Input: part model. Units: mm. Frame: model coordinates. A direction names the side the tool comes from. Coordinates: 2 decimals unless noted, no trailing zeros. Loops run counter-clockwise (first coordinate to the right, second up) from the corner with the lowest first, then second, coordinate; pieces in that order, holes last. Notation, with made-up numbers: (-38.75, 80.5) -> (16.25, 80.5) arc R10 ccw to (16.25, 88.5) -> close; hole circle Ø1 at (35.25, -38). An arc over 180 degrees is marked (long way). Put each result on its own line as item: value. Start each with the question number.
1) Cut plane A-A (y = -8). Return the cut outline in (x, z).
2) Contact query for flat-ended pins moving along their axis: P1, Ø2.5, axis at y = -6.5, z = 94, coming from the -X side; P2, Ø20, axis at x = 64.5, z = 92, coming from the -Y side; P3, Ø2, axis at x = 71.5, y = -8.5, coming from the +Z side; P4, Ø4, axis at y = -8, z = 77, coming from the -X side. Output: stop coordinate, or through.
3) Material intervals for L1, parallel to X at y = -7.4, z = 60; L2, parallel to X at y = -7.75, z = 94; L3, parallel to Y at x = 115.5, z = 38, sorted ascending.
4) Cut plane B-B (z = 69). Return the cut outline in (x, y), plus the area to 3 significant figures.
5) Cut plane C-C (x = 55.5). Return the cut outline in (y, z).
6) Set-up query: faces 1 (the flat face through (61.25, -6, 117)), 2 (the flat face through (64, -7, 112)), 3 (the flat face through (91, -2, 120)). Return all of +Z, -Z, +X, -X, +Y, -Y with unobstructed straight access to the full face (end or side cutting, diameter ignored); none if empty.
7) Pull-direction query (X, two-part tool) for faces 4 (the flat face through (0, -2, 61)), 5 (the flat face through (56, -7, 112)), 6 (the cylindrical face through (61, -8, 1)); classes: pulls with the +X half, pulls with the -X half, needs draft (parallel to the pull), parting line crosses it, or undercut.
from build123d import *

# Parameters (mm, degrees)
F1_DEPTH = 5
F2_DEPTH = 10
F3_R     = 5


with BuildPart() as f1:
    # F0 (on Front) → F1 (new body)
    with BuildSketch(Plane.XZ):
        with BuildLine():
            Line((54, 60), (54, 79.078784))
            ThreePointArc((54, 79.078784), (48.16784, 43.875485), (80, 60))
            ThreePointArc((80, 60), (76.124515, 71.83216), (66, 79.078784))
            Line((66, 79.078784), (66, 60))
            Line((66, 60), (60, 60))
            Line((60, 60), (54, 60))
        make_face()
        with BuildLine():
            ThreePointArc((60, 80), (56.964846, 79.768355), (54, 79.078784))
            Line((54, 79.078784), (54, 60))
            Line((54, 60), (60, 60))
            Line((60, 60), (66, 60))
            Line((66, 60), (66, 79.078784))
            ThreePointArc((66, 79.078784), (63.035154, 79.768355), (60, 80))
        make_face()
        with BuildLine():
            Line((60, 80), (54, 80))
            Line((54, 80), (54, 79.078784))
            ThreePointArc((54, 79.078784), (56.964846, 79.768355), (60, 80))
        make_face()
        with BuildLine():
            Line((66, 79.078784), (66, 80))
            Line((66, 80), (60, 80))
            ThreePointArc((60, 80), (63.035154, 79.768355), (66, 79.078784))
        make_face()
        Polygon((58.75, 112), (54, 112), (54, 80), (60, 80), (66, 80), (66, 112), (61.25, 112), (61.25, 117.5), (58.75, 117.5), align=None)
    extrude(amount=F1_DEPTH)

    # F0 (on Front) → F2 (join)
    with BuildSketch(Plane.XZ):
        with BuildLine():
            Line((0, 120), (0, 0))
            Line((0, 0), (120, 0))
            Line((120, 0), (120, 120))
            Line((120, 120), (66, 120))
            Line((66, 120), (66, 112))
            Line((66, 112), (66, 80))
            Line((66, 80), (66, 79.078784))
            ThreePointArc((66, 79.078784), (76.124515, 71.83216), (80, 60))
            ThreePointArc((80, 60), (48.16784, 43.875485), (54, 79.078784))
            Line((54, 79.078784), (54, 80))
            Line((54, 80), (54, 112))
            Line((54, 112), (54, 120))
            Line((54, 120), (0, 120))
        make_face()
        Polygon((58.75, 120), (54, 120), (54, 112), (58.75, 112), (58.75, 117.5), align=None)
        Polygon((66, 112), (66, 120), (61.25, 120), (61.25, 117.5), (61.25, 112), align=None)
    extrude(amount=F2_DEPTH)

    # F3
    f3_edges = [f1.edges().sort_by_distance(p)[0] for p in [
        (0, -10, 60),
        (60, -10, 0),
        (120, -10, 60),
        (90.625, -10, 120),
        (29.375, -10, 120),
    ]]
    fillet(f3_edges, radius=F3_R)


solid = f1.part
Results found:
1. outline: (1, 1) -> (119, 1) -> (119, 119) -> (61.25, 119) -> (61.25, 112) -> (66, 112) -> (66, 79.08) arc R20 cw (long way) to (54, 79.08) -> (54, 112) -> (58.75, 112) -> (58.75, 119) -> (1, 119) -> close
2. P1: stops at x = 0.01
2. P2: stops at y = -10
2. P3: stops at z = 119.33
2. P4: stops at x = 0.1
3. L1: x = 0.61 to 40, 80 to 119.39
3. L2: x = 0.82 to 54, 66 to 119.18
3. L3: y = -9.97 to 0
4. outline: (0, -5) arc R5 ccw to (5, -10) -> (42.14, -10) -> (42.14, -5) -> (77.86, -5) -> (77.86, -10) -> (115, -10) arc R5 ccw to (120, -5) -> (120, 0) -> (0, 0) -> close
4. area: 1,010 mm2
5. outline: (-10, 5) arc R5 ccw to (-5, 0) -> (0, 0) -> (0, 120) -> (-5, 120) arc R5 ccw to (-10, 115) -> (-10, 112) -> (-5, 112) -> (-5, 40.51) -> (-10, 40.51) -> close
6. face 1: +Z, -Y
6. face 2: -Y
6. face 3: +Z, +X, -X, +Y, -Y
7. face 4: pulls with the -X half
7. face 5: undercut
7. face 6: needs draft
